```python
from build123d import *

# Parameters (mm, degrees)
F3_R     = 5
F4_DEPTH = 2.5019
F5_R     = 5
F6_DEPTH = 2.5


with BuildPart() as f2:
    # F2: sweep along a path in F1
    with BuildLine(Plane.YZ) as f2_path:
        Line((0, -20), (90, -20))
        ThreePointArc((90, -20), (97.0710678119, -22.9289321881), (100, -30))
        Line((100, -30), (100, -70))
        Line((100, -70), (100, -130))
        ThreePointArc((100, -130), (97.0710678119, -137.0710678119), (90, -140))
        Line((90, -140), (0, -140))
    # F0 (on Front) → F2 (sweep)
    with BuildSketch(Plane.XZ):
        with BuildLine():
            Line((10, 20), (0, 20))
            Line((0, 20), (-10, 20))
            Line((-10, 20), (-10, 15))
            Line((-10, 15), (-5.5, 15))
            ThreePointArc((-5.5, 15), (-3.3786796564, 14.1213203436), (-2.5, 12))
            Line((-2.5, 12), (-2.5, 0))
            Line((-2.5, 0), (-2.5, -12))
            ThreePointArc((-2.5, -12), (-3.3786796564, -14.1213203436), (-5.5, -15))
            Line((-5.5, -15), (-10, -15))
            Line((-10, -15), (-10, -20))
            Line((-10, -20), (0, -20))
            Line((0, -20), (10, -20))
            Line((10, -20), (10, -15))
            Line((10, -15), (5.5, -15))
            ThreePointArc((5.5, -15), (3.3786796564, -14.1213203436), (2.5, -12))
            Line((2.5, -12), (2.5, 0))
            Line((2.5, 0), (2.5, 12))
            ThreePointArc((2.5, 12), (3.3786796564, 14.1213203436), (5.5, 15))
            Line((5.5, 15), (10, 15))
            Line((10, 15), (10, 20))
        make_face()
    sweep(path=f2_path.line)

    # F3 (on Right) → F4 (join, symmetric)
    with BuildSketch(Plane.YZ):
        with BuildLine():
            Line((0, 50), (0, 20))
            Line((0, 20), (70, 20))
            Line((70, 20), (34.3131745435, 59.1621407854))
            ThreePointArc((34.3131745435, 59.1621407854), (14.3707898227, 65.0141729122), (0, 50))
        make_face()
        with Locations((19.5303310126, 45.6911520637)):
            Circle(F3_R, mode=Mode.SUBTRACT)
    extrude(amount=F4_DEPTH, both=True)

    # F5 (on Right) → F6 (join, symmetric)
    with BuildSketch(Plane.YZ):
        with BuildLine():
            Line((70, -177.5), (0, -177.5))
            Line((0, -177.5), (0, -207.5))
            ThreePointArc((0, -207.5), (18.9121985963, -231.3187428985), (46.3976711035, -218.2975075473))
            Line((46.3976711035, -218.2975075473), (70, -177.5))
        make_face()
        with Locations((24.4552150904, -207.5)):
            Circle(F5_R, mode=Mode.SUBTRACT)
    extrude(amount=F6_DEPTH, both=True)


solid = f2.part
```
Model file for the job. Use its own axes, mm. A direction names the side the tool comes from. Round coordinates to 2 decimals unless told otherwise and drop trailing zeros. Loops run counter-clockwise (first coordinate to the right, second up) from the corner with the lowest first, then second, coordinate; pieces in that order, holes last. Notation, with made-up numbers: M 1.25,-4.5 L 6.25,-4.5 A8 cw 6.25,1.5 Z; hole C 55,-18.75 d5. An arc over 180 degrees is marked long. Put each result on its own line as item: value. Start each with the question number.
Item 1: Drill centre lines: line 1 along Z through (x, y) = (5.75, 25); line 2 along Z through (x, y) = (-1, 73); line 3 along Y through (x, z) = (-8, -74.5). Where is each one in solid material? Low to high.
Item 2: 3-axis set-ups, long thin cutter, end or side, ignore diameter. For faces 1 (the face through (0, 44, -140)), 2 (the face through (-2.5, 26, -200)), 3 (the face through (2.5, 26, -200)), 4 (the face through (7.781, 122.168, -161.468)), 5 (the face through (2.502, 27, 38)): which of +Z, -Z, +X, -X, +Y, -Y reach the whole face in a straight line?
Item 3: Drop flat-ended pins along their axis: P1, Ø10, axis at x = 3, z = -68.5, coming from the -Y side; P2, Ø13.5, axis at y = 45.5, z = 39.5, coming from the -X side; P3, Ø5, axis at x = 1.5, y = 70.5, coming from the -Z side. Give the stop position or say it passes through.
Item 4: Mould opens along Y. For faces 6 (the face through (7.781, 121.468, 2.168)), 7 (the face through (5, 44, -180)), 8 (the face through (0, 100, -81)) say: released by +Y, released by -Y, zero draft, split by the parting line, or undercut.
Item 5: Cut at A-A (z = -40). List the corners of the cut face in (x, y).
Answer block:
1. line 1: -180 to -175, -145 to -140, -20 to -15, 15 to 20
1. line 2: -180 to -140, -20 to 20
1. line 3: 100 to 105, 135 to 140
2. face 1: +X, -X, -Y
2. face 2: -Z, -X, +Y, -Y
2. face 3: -Z, +X, +Y, -Y
2. face 4: +X
2. face 5: +Z, +X, +Y, -Y
3. P1: y = 100
3. P2: x = -2.5
3. P3: z = -180.96
4. face 6: undercut
4. face 7: zero draft
4. face 8: released by -Y
5. outline: M -10,100 L 10,100 L 10,105 L 5.5,105 A3 cw 2.5,108 L 2.5,132 A3 cw 5.5,135 L 10,135 L 10,140 L -10,140 L -10,135 L -5.5,135 A3 cw -2.5,132 L -2.5,108 A3 cw -5.5,105 L -10,105 Z
